```python
from build123d import *

# Parameters (mm, degrees)
SKETCH_1_R          = 5
EXTRUDE_1_DEPTH     = 2
SKETCH_2_R          = 1.3
CUT_EXTRUDE_1_DEPTH = 2
SKETCH_3_W          = 6
SKETCH_3_H          = 26
SKETCH_3_R          = 1.5
EXTRUDE_2_DEPTH     = 2
FILLET_1_R          = 3
FILLET_2_R          = 2
FILLET_3_R          = 1


with BuildPart() as part:
    # 草图1 → 凸台-拉伸1 (new body)
    with BuildSketch(Plane(origin=(0, 0, 0), x_dir=(1, 0, 0), z_dir=(0, 1, 0))):
        with BuildLine():
            Line((11.180339887, 10), (80, 10))
            Line((80, 10), (80, -10))
            Line((80, -10), (11.180339887, -10))
            ThreePointArc((11.180339887, -10), (0, -15), (-11.180339887, -10))
            Line((-11.180339887, -10), (-80, -10))
            Line((-80, -10), (-80, 10))
            Line((-80, 10), (-11.180339887, 10))
            ThreePointArc((-11.180339887, 10), (0, 15), (11.180339887, 10))
        make_face()
        with Locations(Location((0, 0, 0), (0, 0, 270))):
            Circle(SKETCH_1_R, mode=Mode.SUBTRACT)
    extrude(amount=EXTRUDE_1_DEPTH)

    # 草图2 → 切除-拉伸1 (cut)
    with BuildSketch(Plane(origin=(0, 2, 0), x_dir=(1, 0, 0), z_dir=(0, 1, 0))):
        with Locations(Location((-25, 5, 0), (0, 0, 270))):
            Circle(SKETCH_2_R)
        with Locations(Location((-25, -5, 0), (0, 0, 90))):
            Circle(SKETCH_2_R)
        with Locations(Location((25, -5, 0), (0, 0, 270))):
            Circle(SKETCH_2_R)
        with Locations(Location((25, 5, 0), (0, 0, 90))):
            Circle(SKETCH_2_R)
    extrude(amount=-CUT_EXTRUDE_1_DEPTH, mode=Mode.SUBTRACT)

    # 草图3 → 凸台-拉伸2 (add)
    # profile 1 of 2: a face of its own
    with BuildSketch(Plane(origin=(0, 0, 0), x_dir=(1, 0, 0), z_dir=(0, 1, 0))):
        with Locations((-83, 0)):
            Rectangle(SKETCH_3_W, SKETCH_3_H)
        with Locations(Location((-83, 10, 0), (0, 0, 270))):
            Circle(SKETCH_3_R, mode=Mode.SUBTRACT)
        with Locations(Location((-83, -10, 0), (0, 0, 90))):
            Circle(SKETCH_3_R, mode=Mode.SUBTRACT)
    # profile 2 of 2: a face of its own
    with BuildSketch(Plane(origin=(0, 0, 0), x_dir=(1, 0, 0), z_dir=(0, 1, 0))):
        with Locations((83, 0)):
            Rectangle(SKETCH_3_W, SKETCH_3_H)
        with Locations(Location((83, -10, 0), (0, 0, 270))):
            Circle(SKETCH_3_R, mode=Mode.SUBTRACT)
        with Locations(Location((83, 10, 0), (0, 0, 90))):
            Circle(SKETCH_3_R, mode=Mode.SUBTRACT)
    extrude(amount=EXTRUDE_2_DEPTH)

    # 圆角1
    fillet_1_edges = [part.edges().sort_by_distance(p)[0] for p in [
        (80, 1, 10),
        (80, 1, -10),
        (-80, 1, -10),
        (-80, 1, 10),
    ]]
    fillet(fillet_1_edges, radius=FILLET_1_R - 0.0001)  # a hair under: the kernel refuses the full size

    # 圆角2
    fillet_2_edges = [part.edges().sort_by_distance(p)[0] for p in [
        (-86, 1, 13),
        (-86, 1, -13),
        (86, 1, 13),
        (86, 1, -13),
    ]]
    fillet(fillet_2_edges, radius=FILLET_2_R)

    # 圆角3
    fillet_3_edges = [part.edges().sort_by_distance(p)[0] for p in [
        (-80, 1, 13),
        (-80, 1, -13),
        (80, 1, -13),
        (80, 1, 13),
    ]]
    fillet(fillet_3_edges, radius=FILLET_3_R)


solid = part.part
```
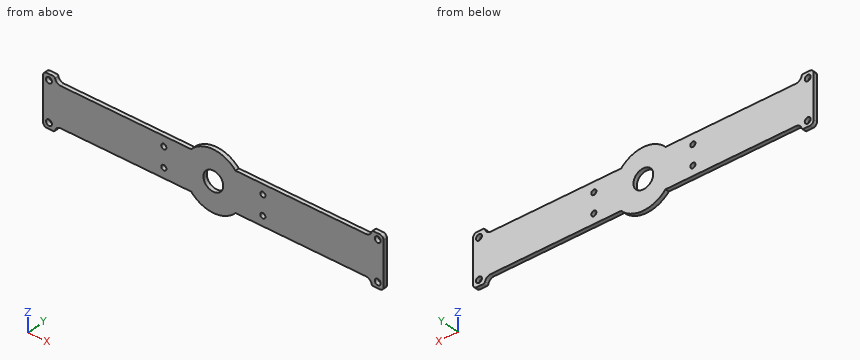
Build history of the part. All positions in model axes, mm. Round coordinates to 2 decimals unless told otherwise and drop trailing zeros. Write each loop counter-clockwise with the first axis right and the second up, starting at its lowest first coordinate (ties: lowest second). Pieces come first, ordered by that corner, then holes. Notation, with made-up numbers: (26.25, -40) -> (44.25, -40) arc R13 ccw to (44.25, -33) -> close; hole circle Ø4 at (32, 20). An arc over 180 degrees is marked (long way). Put each result on its own line as item: value.
Item 1: Slice it at B-B, the plane z = 0. Give the cut face in (x, y), plus the area to 3 significant figures.
Here are the results:
outline: (-86, 0) -> (-5, 0) -> (-5, 2) -> (-86, 2) -> close; (5, 0) -> (86, 0) -> (86, 2) -> (5, 2) -> close
area: 324 mm^2
Item 2: Wall check: probe 1 along Z at (x, y) = (83, 1); probe 2 along X at (y, z) = (0.55, -4.5); probe 3 along X at (y, z) = (0.4, -5.5). Give the ranges that are in metal, low to high. Write a range as from..to.
Here are the results:
probe 1: z = -13..-11.5, -8.5..8.5, 11.5..13
probe 2: x = -86..-26.2, -23.8..-2.18, 2.18..23.8, 26.2..86
probe 3: x = -86..-26.2, -23.8..23.8, 26.2..86
Item 3: Slice it at A-A, the plane x = 0. Give the cut face in (y, z), plus the area to 3 significant figures.
Here are the results:
outline: (0, -15) -> (2, -15) -> (2, -5) -> (0, -5) -> close; (0, 5) -> (2, 5) -> (2, 15) -> (0, 15) -> close
area: 40.0 mm^2
Item 4: Slice it at D-D, the plane x = 68.5. Give the cut face in (y, z), plus the area to 3 significant figures.
Here are the results:
outline: (0, -10) -> (2, -10) -> (2, 10) -> (0, 10) -> close
area: 40.0 mm^2
Item 5: Slice it at C-C, the plane y = 0.4. Count the separate pieces of the cut face and the enclosed holes in it, plus the area to 3 significant figures.
Here are the results:
separate pieces: 1
enclosed holes: 9
area: 3,540 mm^2
Item 6: Flat gauge pins, fed straight in: P1, Ø1.6, axis at x = 25, z = -5, coming from the +Y side; P2, Ø3.5, axis at x = 83, z = -10, coming from the +Y side; P3, Ø0.6, axis at x = -52, y = 0.5, coming from the -Z side; P4, Ø0.6, axis at x = 82.5, y = 1, coming from the +Z side. Where does each tip first touch, or does it go through?
Here are the results:
P1: passes through
P2: stops at y = 2
P3: stops at z = -10
P4: stops at z = 13
